The drawing under review shows one solid part. Ordinate dimensions are in mm from its lowest x, y, z. Give positions to 0.01 mm unless a question says otherwise; leave off trailing zeros. Loops run counter-clockwise (first coordinate to the right, second up) from the corner with the lowest first, then second, coordinate; pieces in that order, holes last. Notation, with made-up numbers: (21, 55) - (55, 55) arc R31 cw to (55, 94) - close; hole circle Ø5 at (67.5, 14). An arc over 180 degrees is marked (long way). Answer as CSV lines item,"result".
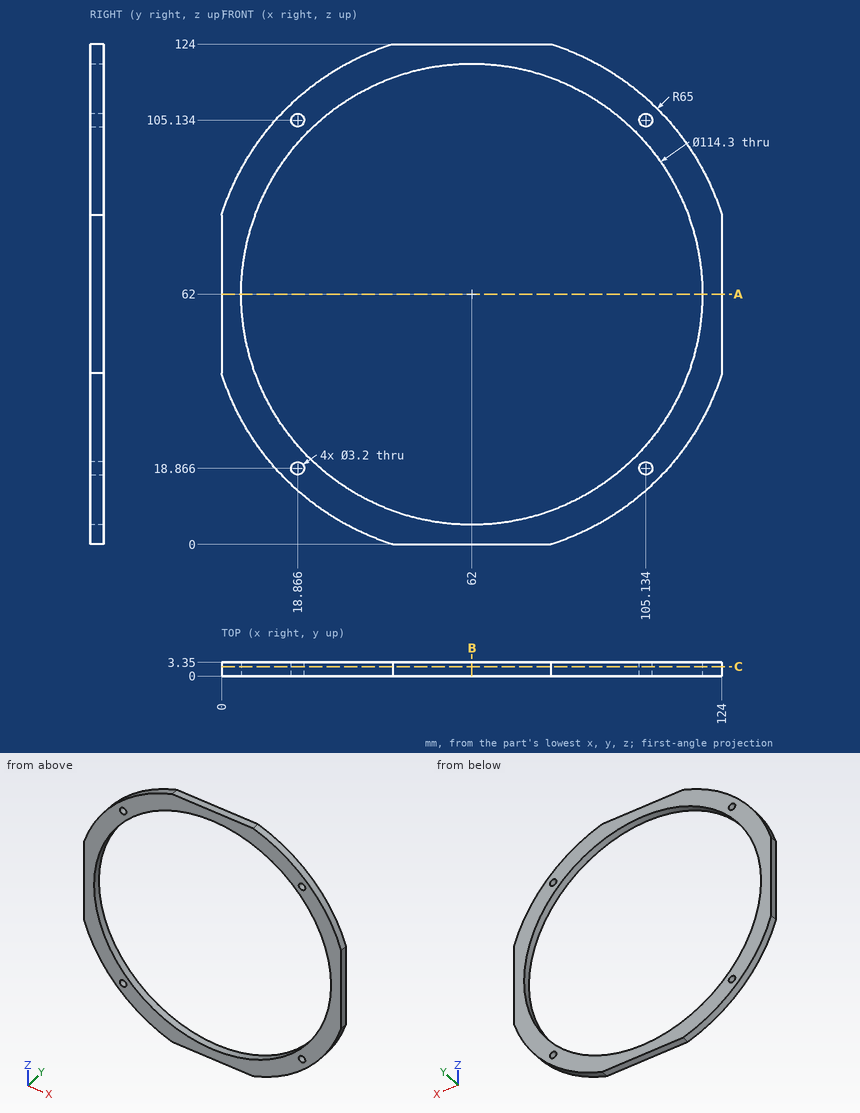
1) Consider section C-C on y = 2.3. Write out the cut boundary in (x, z), and give its area (3 significant figures).
From the geometry:
outline,"(0, 42.48) arc R65 ccw to (42.48, 0) - (81.52, 0) arc R65 ccw to (124, 42.48) - (124, 81.52) arc R65 ccw to (81.52, 124) - (42.48, 124) arc R65 ccw to (0, 81.52) - close; hole circle Ø114.3 at (62, 62); hole circle Ø3.2 at (18.87, 18.87); hole circle Ø3.2 at (18.87, 105.13); hole circle Ø3.2 at (105.13, 18.87); hole circle Ø3.2 at (105.13, 105.13)"
area,"2,670 mm^2"
2) Consider section A-A on z = 62. Write out the cut boundary in (x, y).
From the geometry:
outline,"(0, 0) - (4.85, 0) - (4.85, 3.35) - (0, 3.35) - close; (119.15, 0) - (124, 0) - (124, 3.35) - (119.15, 3.35) - close"
3) Wall thickness on line 1 (X direction, y = 1.5, z = 63.5); line 2 (Z direction, x = 99, y = 1.2) (1 decimal); line 3 (Z direction, x = 99.5, y = 1.8) (1 decimal): over which ranges is each line inside the solid? List them lowest first. Write a range as from..to.
From the geometry:
line 1,"x = 0..4.87, 119.13..124"
line 2,"z = 8.6..18.4, 105.6..115.4"
line 3,"z = 8.9..18.9, 105.1..115.1"
4) Insertion check: P1, Ø3, axis at x = 105.13, z = 18.87, coming from the +Y side (3 decimals); P2, Ø2, axis at y = 1.5, z = 85.5, coming from the +X side. Each pin has a flat end and moves straight along its axis. Give the tip position at first contact, or say it passes through.
From the geometry:
P1,"passes through"
P2,"stops at x = 122.98"
5) Consider section B-B on x = 62. Write out the cut boundary in (y, z), and give its area (3 significant figures).
From the geometry:
outline,"(0, 0) - (3.35, 0) - (3.35, 4.85) - (0, 4.85) - close; (0, 119.15) - (3.35, 119.15) - (3.35, 124) - (0, 124) - close"
area,"32.5 mm^2"
